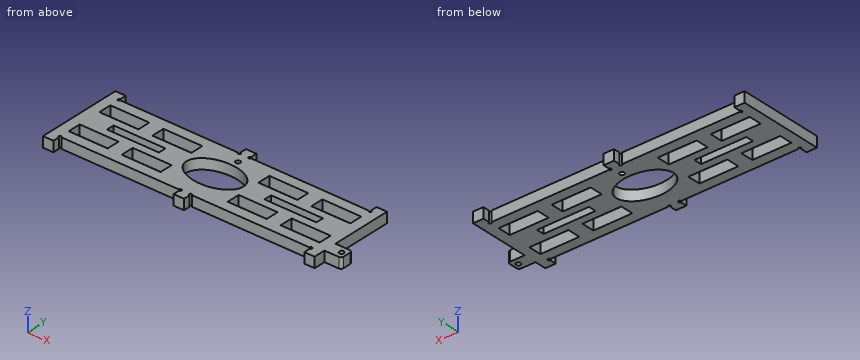
```python
from build123d import *

# Parameters (mm, degrees)
EXTRUDE_2_DEPTH     = 4
SKETCH_3_R          = 0.9
EXTRUDE_3_DEPTH     = 4
SKETCH_4_R          = 0.9
CUT_EXTRUDE_1_DEPTH = 10
SKETCH_5_RX         = 11
SKETCH_5_RY         = 7
SKETCH_5_W          = 15
SKETCH_5_H          = 5
SKETCH_5_W_2        = 20
SKETCH_5_H_2        = 3
CUT_EXTRUDE_2_DEPTH = 10


with BuildPart() as part:
    # 草图2 → 凸台-拉伸2 (new body)
    with BuildSketch(Plane.XY):
        with BuildLine():
            Line((92.360003471, 3.000000026), (46.930000186, 3.000000026))
            ThreePointArc((46.930000186, 3.000000026), (46.076446818, 3.353553971), (46.429999173, 2.499999944))
            Line((46.429999173, 2.499999944), (46.429999173, 0))
            Line((46.429999173, 0), (42.429998517, 0))
            Line((42.429998517, 0), (42.429998517, 2.499999944))
            ThreePointArc((42.429998517, 2.499999944), (42.78355457, 3.35355131), (41.930001229, 3.000000026))
            Line((41.930001229, 3.000000026), (-3.49999981, 3.000000026))
            ThreePointArc((-3.49999981, 3.000000026), (-4.353553201, 3.353553417), (-3.99999981, 2.500000026))
            Line((-3.99999981, 2.500000026), (-3.99999981, 0))
            Line((-3.99999981, 0), (-8, 0))
            Line((-8, 0), (-8, 35.000000149))
            Line((-8, 35.000000149), (-3.99999981, 35.000000149))
            Line((-3.99999981, 35.000000149), (-3.99999981, 32.500000123))
            ThreePointArc((-3.99999981, 32.500000123), (-4.353553201, 31.646446732), (-3.49999981, 32.000000123))
            Line((-3.49999981, 32.000000123), (41.930001229, 32.000000123))
            ThreePointArc((41.930001229, 32.000000123), (42.78355457, 31.646448839), (42.429998517, 32.500000205))
            Line((42.429998517, 32.500000205), (42.429998517, 35.000000149))
            Line((42.429998517, 35.000000149), (46.429999173, 35.000000149))
            Line((46.429999173, 35.000000149), (46.429999173, 32.500000205))
            ThreePointArc((46.429999173, 32.500000205), (46.076446818, 31.646446178), (46.930000186, 32.000000123))
            Line((46.930000186, 32.000000123), (92.360003471, 32.000000123))
            ThreePointArc((92.360003471, 32.000000123), (93.213546668, 31.646450955), (92.8599975, 32.500000123))
            Line((92.8599975, 32.500000123), (92.8599975, 35.000000149))
            Line((92.8599975, 35.000000149), (96.85999769, 35.000000149))
            Line((96.85999769, 35.000000149), (96.85999769, 0))
            Line((96.85999769, 0), (92.8599975, 0))
            Line((92.8599975, 0), (92.8599975, 2.500000026))
            ThreePointArc((92.8599975, 2.500000026), (93.21355089, 3.353553417), (92.360003471, 3.000000026))
        make_face()
    extrude(amount=EXTRUDE_2_DEPTH)


with BuildPart() as body_2:
    # Split Bodies 1: the piece on the far side of the plane
    add(part.part)
    split(bisect_by=Plane.YZ.offset(48.429999172), keep=Keep.BOTTOM)


with BuildPart() as part_1:
    add(part.part)

    # Split Bodies 1
    split(bisect_by=Plane.YZ.offset(48.429999172), keep=Keep.TOP)


with BuildPart() as part_2:
    # Move Body 1: moved
    add(part_1.part.moved(Location((-0.1, 0, 0))))


with BuildPart() as body_3:
    # Split Bodies 2: the piece on the far side of the plane
    add(body_2.part)
    split(bisect_by=Plane(origin=(40.429998517, 0, 0), x_dir=(0, -1, 0), z_dir=(-1, 0, 0)), keep=Keep.BOTTOM)


with BuildPart() as body_2_1:
    add(body_2.part)

    # Split Bodies 2
    split(bisect_by=Plane(origin=(40.429998517, 0, 0), x_dir=(0, -1, 0), z_dir=(-1, 0, 0)), keep=Keep.TOP)


with BuildPart() as body_2_2:
    # Move Body 2: moved
    add(body_2_1.part.moved(Location((0.1, 0, 0))))


with BuildPart() as part_3:
    add(part_2.part)

    # Combine 2: union body 3, body 2
    add(body_3.part)
    add(body_2_2.part)


with BuildPart() as body_2_2_1:
    # Split Bodies 3: the piece on the far side of the plane
    add(part_3.part)
    split(bisect_by=Plane(origin=(0, 27.000000123, 0), x_dir=(1, 0, 0), z_dir=(0, 1, 0)), keep=Keep.BOTTOM)


with BuildPart() as part_4:
    add(part_3.part)

    # Split Bodies 3
    split(bisect_by=Plane(origin=(0, 27.000000123, 0), x_dir=(1, 0, 0), z_dir=(0, 1, 0)), keep=Keep.TOP)


with BuildPart() as part_5:
    # Move Body 3: moved
    add(part_4.part.moved(Location((0, -2, 0))))

    # Combine 3: union body 2 2
    add(body_2_2_1.part)

    # 草图3 → 凸台-拉伸3 (add)
    with BuildSketch(Plane(origin=(0, 0, 0), x_dir=(-1, 0, 0), z_dir=(0, 0, -1))):
        with BuildLine():
            Line((-102.25999769, 9.500000075), (-96.75999769, 9.500000075))
            Line((-96.75999769, 9.500000075), (-96.75999769, 4.500000075))
            Line((-96.75999769, 4.500000075), (-102.25999769, 4.500000074))
            ThreePointArc((-102.25999769, 4.500000074), (-102.967104471, 4.792893293), (-103.25999769, 5.500000074))
            Line((-103.25999769, 5.500000074), (-103.25999769, 8.500000075))
            ThreePointArc((-103.25999769, 8.500000075), (-102.967104471, 9.207106856), (-102.25999769, 9.500000075))
        make_face()
        with Locations((-101.25999769, 7.000000075)):
            Circle(SKETCH_3_R, mode=Mode.SUBTRACT)
    extrude(amount=-EXTRUDE_3_DEPTH)

    # 草图4 → 切除-拉伸1 (cut)
    with BuildSketch(Plane(origin=(0, 0, 0), x_dir=(-1, 0, 0), z_dir=(0, 0, -1))):
        with Locations((-45.25999769, 26.000000075)):
            Circle(SKETCH_4_R)
    extrude(amount=-CUT_EXTRUDE_1_DEPTH, mode=Mode.SUBTRACT)

    # 草图5 → 切除-拉伸2 (cut)
    with BuildSketch(Plane(origin=(0, 0, 0), x_dir=(-1, 0, 0), z_dir=(0, 0, -1))):
        with Locations((-44.429998845, 16.500000074)):
            Ellipse(SKETCH_5_RX, SKETCH_5_RY)
        with Locations((-85.25999769, 23.500000123)):
            Rectangle(SKETCH_5_W, SKETCH_5_H)
        with Locations((-64.844998267, 23.500000123)):
            Rectangle(SKETCH_5_W, SKETCH_5_H)
        with Locations((-24.014999422, 23.500000123)):
            Rectangle(SKETCH_5_W, SKETCH_5_H)
        with Locations((-3.6, 23.500000123)):
            Rectangle(SKETCH_5_W, SKETCH_5_H)
        with Locations((-3.6, 9.500000026)):
            Rectangle(SKETCH_5_W, SKETCH_5_H)
        with Locations((-24.014999422, 9.500000026)):
            Rectangle(SKETCH_5_W, SKETCH_5_H)
        with Locations((-64.844998267, 9.500000026)):
            Rectangle(SKETCH_5_W, SKETCH_5_H)
        with Locations((-85.25999769, 9.500000026)):
            Rectangle(SKETCH_5_W, SKETCH_5_H)
        with Locations((-74.75999769, 16.500000123)):
            Rectangle(SKETCH_5_W_2, SKETCH_5_H_2)
        with Locations((-14.1, 16.500000123)):
            Rectangle(SKETCH_5_W_2, SKETCH_5_H_2)
    extrude(amount=-CUT_EXTRUDE_2_DEPTH, mode=Mode.SUBTRACT)


solid = part_5.part
```
Model file for the job. Use its own axes, mm. Give positions to 0.01 mm unless a question says otherwise; leave off trailing zeros. Order: outer loops, then holes, each group sorted by start corner. A loop starts at its lowest first (then second) coordinate and runs counter-clockwise, first axis right, second up.
1) Saw through at A-A, the plane x = 88.5. Write the cut outline in (y, z).
2) Wall check: probe 1 along Y at (x, z) = (23, 1.1); probe 2 along Y at (x, z) = (64.5, 2.8); probe 3 along X at (y, z) = (24.5, 2.25) (3 decimals). Give the ranges that are in metal, low to high.
3) Pin check, flat tips, straight feed: pin 1 (1.2 mm diameter, centred on x = 99.5, z = 2, fed in from +Y); pin 2 (2 mm diameter, centred on x = 14.5, z = 2.5, fed in from -Y); pin 3 (2 mm diameter, centred on x = 5.5, z = 2, fed in from +Y). Stop position of each tip, or through.
4) Saw through at C-C, the plane y = 22.5. Count the separate pieces of the cut face and the enclosed holes in it, then the cut area to 3 significant figures.
5) Saw through at B-B, the plane x = 73.5. Write the cut outline in (y, z), then the cut area to 3 significant figures.
Computed:
1. outline: (3, 0) - (7, 0) - (7, 4) - (3, 4) - close; (12, 0) - (21, 0) - (21, 4) - (12, 4) - close; (26, 0) - (30, 0) - (30, 4) - (26, 4) - close
2. probe 1: y = 3 to 7, 12 to 15, 18 to 21, 26 to 30
2. probe 2: y = 3 to 7, 12 to 21, 26 to 30
2. probe 3: x = -7.9 to -3.9, 11.1 to 16.515, 31.515 to 57.345, 72.345 to 77.76, 92.76 to 96.76
3. pin 1: stops at y = 9.5
3. pin 2: stops at y = 3
3. pin 3: stops at y = 30
4. separate pieces: 6
4. enclosed holes: 0
4. area: 133 mm2
5. outline: (3, 0) - (15, 0) - (15, 4) - (3, 4) - close; (18, 0) - (30, 0) - (30, 4) - (18, 4) - close
5. area: 96.0 mm2
